```python
from build123d import *

# Parameters (mm, degrees)
SKETCH_W        = 94
SKETCH_H        = 83
PAD_DEPTH       = 6
SKETCH001_R     = 2.25
POCKET_DEPTH    = 6.001
FILLET_R        = 3
FILLET001_R     = 3
FILLET002_R     = 3
FILLET003_R     = 3
SKETCH002_W     = 5
SKETCH002_H     = 20
POCKET001_DEPTH = 6.001


with BuildPart() as part:
    # Sketch → Pad (new body)
    with BuildSketch(Plane.XY):
        with Locations((47, 41.5)):
            Rectangle(SKETCH_W, SKETCH_H)
    extrude(amount=PAD_DEPTH)

    # Sketch001 (on Face6 of Pad) → Pocket (cut, through all)
    with BuildSketch(Plane.XY.offset(6)):
        with Locations((4, 79)):
            Circle(SKETCH001_R)
        with Locations((90, 79)):
            Circle(SKETCH001_R)
        with Locations((90, 4)):
            Circle(SKETCH001_R)
        with Locations((4, 4)):
            Circle(SKETCH001_R)
    extrude(amount=-POCKET_DEPTH, mode=Mode.SUBTRACT)

    # Fillet
    fillet_edges = [part.edges().sort_by_distance(p)[0] for p in [
        (94, 0, 3),
    ]]
    fillet(fillet_edges, radius=FILLET_R)

    # Fillet001
    fillet001_edges = [part.edges().sort_by_distance(p)[0] for p in [
        (94, 83, 3),
    ]]
    fillet(fillet001_edges, radius=FILLET001_R)

    # Fillet002
    fillet002_edges = [part.edges().sort_by_distance(p)[0] for p in [
        (0, 83, 3),
    ]]
    fillet(fillet002_edges, radius=FILLET002_R)

    # Fillet003
    fillet003_edges = [part.edges().sort_by_distance(p)[0] for p in [
        (0, 0, 3),
    ]]
    fillet(fillet003_edges, radius=FILLET003_R)

    # Sketch002 (on Face14 of Fillet003) → Pocket001 (cut, through all)
    with BuildSketch(Plane.XY.offset(6)):
        with Locations((11.5, 39)):
            Rectangle(SKETCH002_W, SKETCH002_H)
    extrude(amount=-POCKET001_DEPTH, mode=Mode.SUBTRACT)


solid = part.part
```
Model file for the job. Use its own axes, mm. A direction names the side the tool comes from. Give positions to 0.01 mm unless a question says otherwise; leave off trailing zeros. Order: outer loops, then holes, each group sorted by start corner. A loop starts at its lowest first (then second) coordinate and runs counter-clockwise, first axis right, second up.
1) Mould opens along Y. For faces 1 (the flat face through (9, 39, 3)), 2 (the cylindrical face through (93.14, 82.1, 3.04)), 3 (the flat face through (46, 42, 6)) say: +Y half, -Y half, draft (parallel to the pull), parting line (faces both ways), or undercut.
2) Pin check, flat tips, straight feed: pin 1 (7 mm diameter, centred on x = 90, y = 4, fed in from -Z); pin 2 (4 mm diameter, centred on x = 90, y = 79, fed in from +Z). Stop position of each tip, or through.
3) Wall check: probe 1 along Y at (x, z) = (90, 1.8); probe 2 along X at (y, z) = (47.5, 2.1); probe 3 along Y at (x, z) = (5.5, 3.5). Give the ranges that are in metal, low to high.
4) Saw through at A-A, the plane y = 46. Write the cut outline in (x, z).
5) 3-axis set-ups, long thin cutter, end or side, ignore diameter. For faces 4 (the flat face through (14, 39, 3)), 5 (the cylindrical face through (0.9, 82.14, 3.04)): which of +Z, -Z, +X, -X, +Y, -Y reach the whole face in a straight line?
Computed:
1. face 1: undercut
1. face 2: +Y half
1. face 3: draft
2. pin 1: stops at z = 0
2. pin 2: passes through
3. probe 1: y = 0 to 1.75, 6.25 to 76.75, 81.25 to 83
3. probe 2: x = 0 to 9, 14 to 94
3. probe 3: y = 0 to 2.32, 5.68 to 77.32, 80.68 to 83
4. outline: (0, 0) - (9, 0) - (9, 6) - (0, 6) - close; (14, 0) - (94, 0) - (94, 6) - (14, 6) - close
5. face 4: +Z, -Z
5. face 5: +Z, -Z, -X, +Y
